Autodesk Inventor part; units mm, degrees
ref_plane "Work Plane12" through (28.1397, 19.0829, 79) normal (-0.589, -0.8081, 0) x (-0.8081, 0.589, 0)
ref_plane "Work Plane13" through (0, 24.8688, 0) normal (1, 0, 0) x (0, 0, 1)
ref_plane "YZ Plane" through (0, 0, 0) normal (1, 0, 0) x (0, 1, 0)
sketch "Sketch8" plane through (0, 0, 0) normal (0, 0, 1) x (1, 0, 0)
  arc A0 (23.5572, 24.5165) -> (-23.5572, 24.5165) centre (0, 0) ccw
  arc A1 (25, 24.4949) -> (-25, 24.4949) centre (0, 0) ccw
  line L0 (-23.5572, 24.5165) -> (-25, 24.4949)
  line L1 (-24.431, 23.6769) -> (-22.7081, 25.3323) construction
  line L2 (22.7844, 25.2591) -> (24.3419, 23.7625) construction
  line L3 (23.5572, 24.5165) -> (25, 24.4949)
  line L4 (-25, 24.4949) -> (25, 24.4949) construction
  dimension "d88" = 34
  dimension "d89" = 35
  dimension "d90" = 0
  dimension "d91" = 137
  dimension "d92" = 0
  dimension "d93" = 137
  dimension "d98" = 50
extrude "Extrusion5" add sketch "Sketch8" along normal blind 79
sketch "Sketch19" plane through (0, 0, 79) normal (0, 0, 1) x (1, 0, 0)
  line L0 (-25, 24.4949) -> (-23.5572, 24.5165) construction
  line L1 (-22.2755, 25.021) -> (-7.4699, 32.6566) construction
  arc A0 (22.2755, 25.021) -> (-22.2755, 25.021) centre (0, 0) ccw construction
  dimension "d162" = 32.448
sketch "Sketch22" plane through (0, 0, 79) normal (0, 0, 1) x (1, 0, 0)
  line L0 (0, 0) -> (23.9071, 24.8806) construction
  line L1 (0, 0) -> (31.302, 21.2274) construction
  arc A0 (23.5572, 24.5165) -> (-23.5572, 24.5165) centre (0, 0) ccw construction
  arc A1 (29.7973, 16.3744) -> (23.5572, 24.5165) centre (0, 0) ccw construction
  line L2 (28.1397, 19.0829) -> (9.553, 32.6304) construction
  point P0 (19.5664, 25.3318)
  dimension "d175" = 12
  dimension "d176" = 23
  dimension "d177" = 0
  dimension "d178" = 10.609
sketch "Sketch23" plane through (0, 0, 0) normal (0, 0, -1) x (-1, 0, 0)
  arc A0 (23.5572, 24.5165) -> (-23.5572, 24.5165) centre (0, 0) ccw
  line L0 (0, 0) -> (-23.5572, 24.5165) construction
  line L1 (0, 0) -> (-31.0154, 21.0331) construction
  arc A1 (-23.5572, 24.5165) -> (-29.6271, 16.6805) centre (0, 0) ccw construction
  line L2 (-28.1397, 19.0829) -> (-9.553, 32.6304) construction
  dimension "d179" = 12
  dimension "d180" = 23
ref_plane "Work Plane12" through (28.1397, 19.0829, 79) normal (-0.589, -0.8081, 0) x (-0.8081, 0.589, 0)
sketch "Sketch24" plane through (28.1397, 19.0829, 79) normal (-0.589, -0.8081, 0) x (-0.8081, 0.589, 0)
  line L0 (6.9037, 79) -> (6.9037, 0)
  line L1 (44.9777, 0) -> (6.9037, 0)
  line L2 (44.9777, 79) -> (6.9037, 79)
  point P0 (11.5, 79)
  point P1 (10.4037, 75.5)
  point P2 (10.4037, 4)
  dimension "d181" = 3.5
  dimension "d182" = 4
  dimension "d183" = 3.5
  dimension "d184" = 3.5
hole "Hole11" at (19.7323, 25.2109, 3.5) at (19.7323, 25.2109, 75) direction (0.589, 0.8081, 0) diameter 2 end through all
ref_plane "Work Plane13" through (0, 24.8688, 0) normal (1, 0, 0) x (0, 0, 1)
mirror "Mirror2" about plane through (0, 24.8688, 0) normal (1, 0, 0) of "Hole11"
properties part number "Electronics Door"
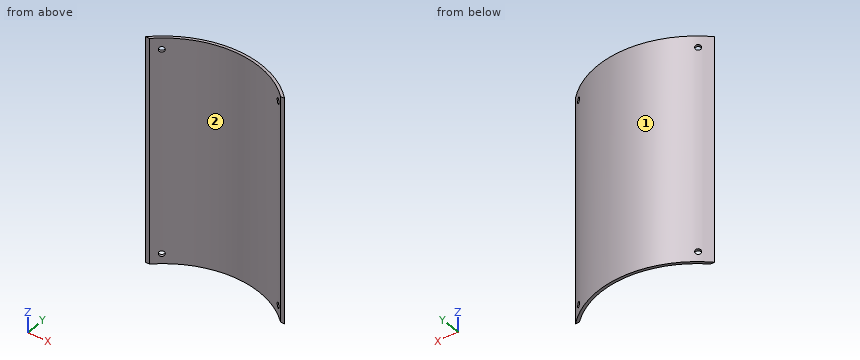
Work out the finished part from the listing and answer in its coordinate system (mm). Face numbers are marked on the shaded views. Give positions to 0.01 mm unless a question says otherwise; leave off trailing zeros. Loops run counter-clockwise (first coordinate to the right, second up) from the corner with the lowest first, then second, coordinate; pieces in that order, holes last. Notation, with made-up numbers: (50.25, 86.25) -> (96.25, 86.25) arc R12 cw to (96.25, 106.25) -> close; hole circle Ø9 at (18, -4.5). An arc over 180 degrees is marked (long way). Use a Markdown table: item, result. Add a question column.
1. Section A-A on y = 31.5 is taken. Determine the outline of the cut face in (x, z), and give its area (3 significant figures).
2. Flat-ended cylindrical pins translate along their axes: pin 1 Ø4 at (y, z) = (32.5, 46.5) entering from -X; pin 2 Ø1 at (x, z) = (7, 16.5) entering from -Y; pin 3 Ø2 at (x, z) = (13.5, 53) entering from -Y. Find the tip coordinate at first contact, or state that the pin passes through.
3. Find the intervals of material crossed by probe 1 along X at (y, z) = (30.5, 40) (3 decimals); probe 2 along X at (y, z) = (30.75, 50); probe 3 along Y at (x, z) = (7.5, 70), in increasing order.
4. Section B-B on z = 57.5 is taken. Determine the outline of the cut face in (x, y), and give its area (3 significant figures).
5. Determine the mould class of the marked faces 1 and 2 for opening direction X: released by +X, released by -X, zero draft, split by the parting line, or undercut.
6. Section C-C on x = -15.5 is taken. Determine the outline of the cut face in (y, z), and give its area (3 significant figures).
Results below:
| question | item | result |
|---|---|---|
| 1 | outline | (-15.26, 0) -> (-12.8, 0) -> (-12.8, 79) -> (-15.26, 79) -> close; (12.8, 0) -> (15.26, 0) -> (15.26, 79) -> (12.8, 79) -> close |
| 1 | area | 389 mm^2 |
| 2 | pin 1 | stops at x = -17.17 |
| 2 | pin 2 | stops at y = 33.16 |
| 2 | pin 3 | stops at y = 30.75 |
| 3 | probe 1 | x = -17.168 to -15.025, 15.025 to 17.168 |
| 3 | probe 2 | x = -16.72 to -14.51, 14.51 to 16.72 |
| 3 | probe 3 | y = 33.16 to 34.19 |
| 4 | outline | (-25, 24.49) -> (-23.56, 24.52) arc R34 cw to (23.56, 24.52) -> (25, 24.49) arc R35 ccw to start |
| 4 | area | 53.9 mm^2 |
| 5 | face 1 | split by the parting line |
| 5 | face 2 | undercut |
| 6 | outline | (30.26, 0) -> (31.38, 0) -> (31.38, 79) -> (30.26, 79) -> close |
| 6 | area | 88.4 mm^2 |
